```python
from build123d import *

# Parameters (mm, degrees)
EXTRUDE_1_DEPTH = 12.5
CHAMFER_1_SIZE  = 15


with BuildPart() as part:
    # Эскиз1 → Бобышка-Вытянуть1 (new body, symmetric)
    with BuildSketch(Plane.XY):
        Polygon((0, 300), (-25, 300), (-125, 40), (-125, 0), (0, 0), align=None)
    extrude(amount=EXTRUDE_1_DEPTH, both=True)

    # Фаска1
    chamfer_1_edges = [part.edges().sort_by_distance(p)[0] for p in [
        (0, 0, 0),
    ]]
    chamfer(chamfer_1_edges, length=CHAMFER_1_SIZE)


solid = part.part
```
Geometry: final body of the model. Coordinates: model frame, mm. Round coordinates to 2 decimals unless told otherwise and drop trailing zeros. Write each loop counter-clockwise with the first axis right and the second up, starting at its lowest first coordinate (ties: lowest second). Pieces come first, ordered by that corner, then holes. Notation, with made-up numbers: M 36.25,68.5 L 71.25,68.5 A31 cw 71.25,93.5 Z; hole C -32,8.25 d5. An arc over 180 degrees is marked long. Answer in a Markdown table with one row per item. Add a question column.
(1) Cut plane B-B, the plane x = -52. Return the cut outline in (y, z), then the cut area to 4 significant figures.
(2) Contact query for flat-ended pins moving along their axis: pin 1 (5 mm diameter, centred on y = 134, z = 7.5, fed in from -X); pin 2 (8 mm diameter, centred on y = 160.5, z = -4.5, fed in from -X); pin 3 (6 mm diameter, centred on y = 63.5, z = 2, fed in from -X). Output: stop coordinate, or through.
(3) Cut plane C-C, the plane y = 222. Return the cut outline in (x, z).
(4) Cut plane A-A, the plane z = -0.75. Return the cut outline in (x, y).
(5) Ray query, L1, parallel to X at y = 212, z = -3.5; L2, parallel to X at y = 275.5, z = 8; L3, parallel to Y at x = -13.5, z = -3.5. Return the intervals inside material, ascending.
Established:
| question | item | result |
|---|---|---|
| 1 | outline | M 0,-12.5 L 229.8,-12.5 L 229.8,12.5 L 0,12.5 Z |
| 1 | area | 5,745 mm² |
| 2 | pin 1 | x = -89.81 |
| 2 | pin 2 | x = -80.19 |
| 2 | pin 3 | x = -117.12 |
| 3 | outline | M -55,-12.5 L 0,-12.5 L 0,12.5 L -55,12.5 Z |
| 4 | outline | M -125,0 L -15,0 L 0,15 L 0,300 L -25,300 L -125,40 Z |
| 5 | L1 | -58.85 to 0 |
| 5 | L2 | -34.42 to 0 |
| 5 | L3 | 1.5 to 300 |
